Geometry: see drawing. Coordinates: mm, zero at the bounding-box minimum. A direction names the side the tool comes from. Give positions to 0.01 mm unless a question says otherwise; leave off trailing zeros. Loops run counter-clockwise (first coordinate to the right, second up) from the corner with the lowest first, then second, coordinate; pieces in that order, holes last. Notation, with made-up numbers: M 3,72.25 L 18,72.25 A11 ccw 18,82.25 Z; hole C 73,21 d9. An arc over 180 degrees is marked long. Put each result on its own line as item: value.
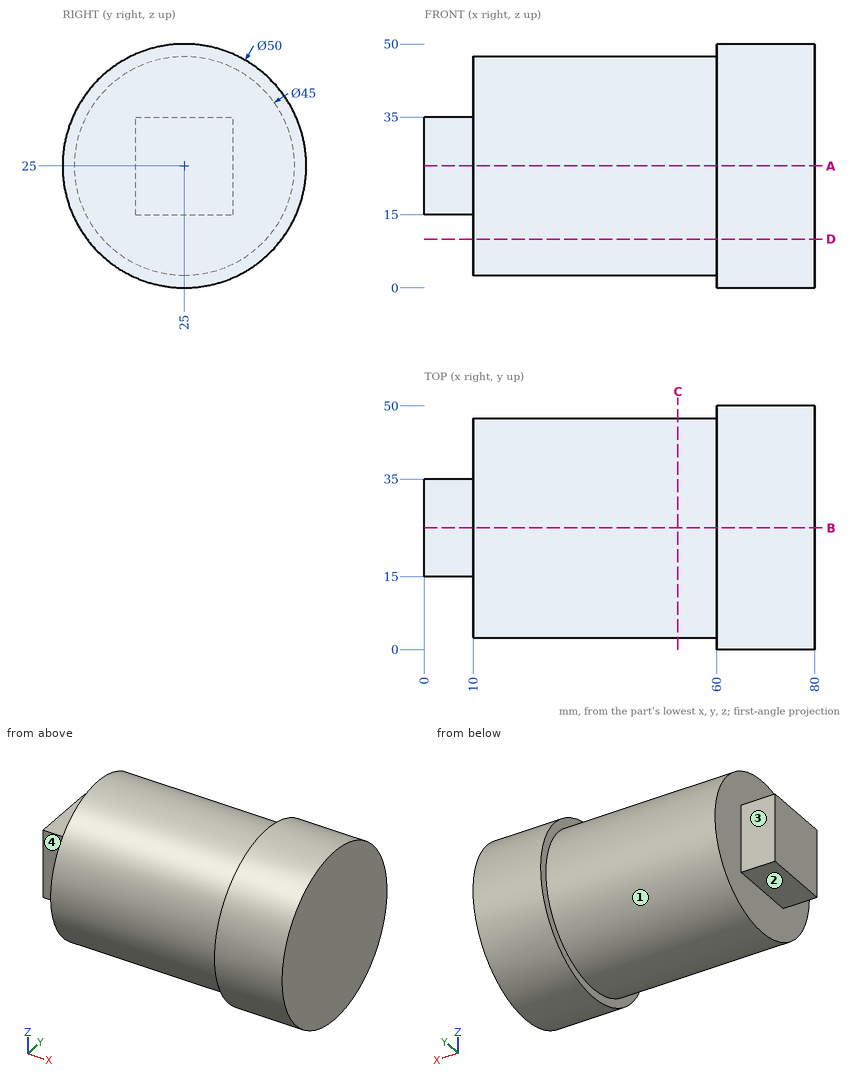
Item 1: Section D-D on z = 10. Output: boundary loops of the cut face in (x, y).
Output values:
outline: M 10,8.23 L 60,8.23 L 60,5 L 80,5 L 80,45 L 60,45 L 60,41.77 L 10,41.77 Z
Item 2: Section C-C on x = 52. Output: boundary loops of the cut face in (y, z).
Output values:
outline: C 25,25 d45
Item 3: Line query: probe 1 along X at (y, z) = (42, 30); probe 2 along Z at (x, y) = (28.5, 24.5); probe 3 along X at (y, z) = (41, 42.5). Output: solid intervals per line, ascending. Write a range as [from, to].
Output values:
probe 1: [10, 80]
probe 2: [2.51, 47.49]
probe 3: [60, 80]
Item 4: Pin query (flat end, axial travel): pin 1 Ø2 at (x, y) = (11, 23) entering from -Z; pin 2 Ø11 at (x, y) = (3.5, 24) entering from -Z; pin 3 Ø4 at (x, z) = (41.5, 19.5) entering from +Y. Return the tip coordinate at first contact, or that it passes through.
Output values:
pin 1: z = 2.52
pin 2: z = 15
pin 3: y = 47.23
Item 5: Set-up query: the marked faces 1, 2, 3 and 4. Return all of +Z, -Z, +X, -X, +Y, -Y with unobstructed straight access to the full face (end or side cutting, diameter ignored); none if empty.
Output values:
face 1: -X
face 2: -Z, -X, +Y, -Y
face 3: +Z, -Z, -X, +Y
face 4: +Z, -Z, -X, -Y
Item 6: Section A-A on z = 25. Output: boundary loops of the cut face in (x, y), then the cut area to 3 significant figures.
Output values:
outline: M 0,15 L 10,15 L 10,2.5 L 60,2.5 L 60,0 L 80,0 L 80,50 L 60,50 L 60,47.5 L 10,47.5 L 10,35 L 0,35 Z
area: 3,450 mm²
